Autodesk Fusion 360 part; units mm, degrees
sketch "Sketch1" plane through (0, 0, 0) normal (0, 0, 1) x (1, 0, 0)
  line L0 (-50, 0) -> (0, 0)
  line L1 (25, 25) -> (0, 0)
  line L2 (-50, 0) -> (-50, 140)
  line L3 (21.9831, 108.8475) -> (-62.7657, 108.8475)
  line L4 (-50, 108.8475) -> (-62.7657, 108.8475)
  line L5 (25, 25) -> (25, 110)
  line L6 (21.9831, 108.8475) -> (25, 108.8475)
extrude "Extrude1" add sketch "Sketch1" along normal blind 25
sketch "Sketch2" plane through (0, 0, 25) normal (0, 0, 1) x (-1, 0, 0)
  line L0 (-25, -108.8475) -> (50, -108.8475)
  line L1 (50, -108.8475) -> (50, 0)
  line L2 (50, 0) -> (0, 0)
  line L3 (0, 0) -> (-25, -25)
  line L4 (-25, -25) -> (-25, -108.8475)
sketch "Sketch3" plane through (0, 0, 25) normal (0, 0, 1) x (-1, 0, 0)
  line L0 (-10, -90) -> (-25, -97)
  line L1 (-25, -108.8475) -> (-25, -97)
  line L2 (-10, -90) -> (50, -90)
  line L3 (19.1012, -90) -> (19.1012, -70)
  line L4 (19.1012, -70) -> (40, -20)
  line L5 (40, -20) -> (40, 0)
  line L6 (40, 0) -> (50, 0)
  line L7 (50, 0) -> (50, -108.8475)
  line L8 (50, -90) -> (50, -108.8475)
  line L9 (-25, -97) -> (-25, -108.8475)
  line L10 (50, -108.8475) -> (50, -90)
  point P0 (-25, -108.8475)
  point P1 (50, 0)
  point P2 (50, -108.8475)
extrude "Extrude2" add sketch "Sketch3" along normal blind 16
sketch "Sketch4" plane through (0, 0, 25) normal (0, 0, 1) x (-1, 0, 0)
  line L0 (-10, -90) -> (-25, -100)
  line L1 (-25, -108.8475) -> (-25, -100)
  line L2 (-25, -108.8475) -> (50, -108.8475)
  line L3 (50, -108.8475) -> (50, -90)
  line L4 (50, -90) -> (-10, -90)
  point P0 (-25, -108.8475)
  point P1 (50, -108.8475)
extrude "Extrude3" add sketch "Sketch4" along normal blind 25
sketch "Sketch5" plane through (0, 0, 41) normal (0, 0, 1) x (-1, 0, 0)
  line L0 (19.1012, -90) -> (50, -90)
  line L1 (50, -90) -> (50, 0)
  line L2 (50, 0) -> (40, 0)
  line L3 (40, 0) -> (40, -20)
  line L4 (40, -20) -> (19.1012, -70)
  line L5 (19.1012, -70) -> (19.1012, -90)
  circle A0 centre (35, -75) radius 5
extrude "Extrude4" cut sketch "Sketch5" against normal blind 41 contours A0
sketch "Sketch6" plane through (0, 90, 0) normal (0, -1, 0) x (1, 0, 0)
  line L0 (-50, 41) -> (-19.1012, 41)
  line L1 (-19.1012, 41) -> (-19.1012, 25)
  line L2 (-19.1012, 25) -> (10, 25)
  line L3 (10, 25) -> (10, 50)
  line L4 (10, 50) -> (-50, 50)
  line L5 (-50, 50) -> (-50, 41)
  circle A0 centre (-10, 35) radius 5
  dimension "d11" = 10
extrude "Extrude5" cut sketch "Sketch6" against normal blind 25 contours A0
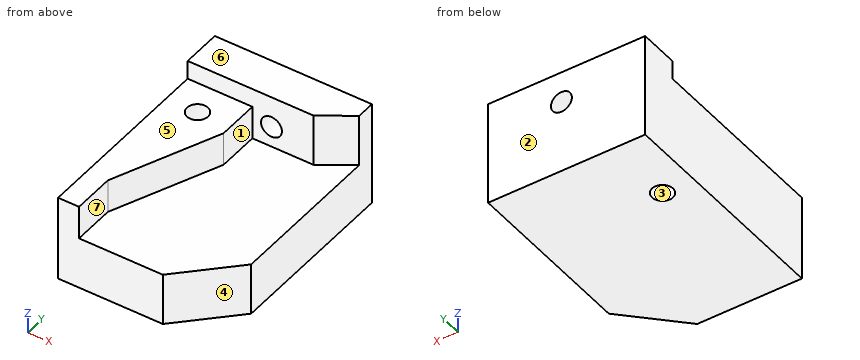
Read the model definition and answer for the solid it produces. Units are mm, in the model's axes. Face numbers are marked on the shaded views. A direction names the side the tool comes from. Round coordinates to 2 decimals unless told otherwise and drop trailing zeros. Loops run counter-clockwise (first coordinate to the right, second up) from the corner with the lowest first, then second, coordinate; pieces in that order, holes last. Notation, with made-up numbers: (-18.5, 6) -> (-7.5, 6) arc R35 cw to (-7.5, 43) -> close; hole circle Ø2 at (17, -3). An arc over 180 degrees is marked (long way). One line per item, written item: value.
1) The mould has two halves that part along Y. Classify the marked faces 1, 2, 3 and 4: pulls with the +Y half, pulls with the -Y half, needs draft (parallel to the pull), parting line crosses it, or undercut.
Answer list:
face 1: needs draft
face 2: pulls with the +Y half
face 3: undercut
face 4: pulls with the -Y half
2) For the marked faces 5, 6 and 7, determine the directions among +Z, -Z, +X, -X, +Y, -Y from which every point of the face is accessible in a straight line to the end or side of a thin tool.
Answer list:
face 5: +Z, +X, -X, -Y
face 6: +Z, +X, -X, +Y, -Y
face 7: +Z, +X, -Y
3) Consider L1, parallel to Y at x = -35, z = 23; L2, parallel to X at y = 75, z = 32; L3, parallel to Z at x = -10, y = 98. Determine where each line is inside the solid, lowest interval first. Write a range as [from, to].
Answer list:
L1: y = [0, 70], [80, 108.85]
L2: x = [-50, -40], [-30, -19.1]
L3: z = [0, 30], [40, 50]
4) A cutting plane is placed at B-B (x = -10). Determine the outline of the cut face in (y, z).
Answer list:
outline: (0, 0) -> (108.85, 0) -> (108.85, 30) -> (90, 30) -> (90, 25) -> (0, 25) -> close; (90, 40) -> (108.85, 40) -> (108.85, 50) -> (90, 50) -> close
5) A cutting plane is placed at C-C (z = 6.5). Determine the outline of the cut face in (x, y).
Answer list:
outline: (-50, 0) -> (0, 0) -> (25, 25) -> (25, 108.85) -> (-50, 108.85) -> close; hole circle Ø10 at (-35, 75)
6) A cutting plane is placed at D-D (x = 3). Determine the outline of the cut face in (y, z).
Answer list:
outline: (3, 0) -> (108.85, 0) -> (108.85, 50) -> (90, 50) -> (90, 25) -> (3, 25) -> close
7) Flat-ended cylindrical pins translate along their axes: P1, Ø6, axis at x = -23, y = 73.5, coming from the +Z side; P2, Ø1.5, axis at x = -18, y = 51.5, coming from the +Z side; P3, Ø10, axis at x = -19.5, y = 21.5, coming from the -Z side; P4, Ø13, axis at y = 76.5, z = 35, coming from the +X side. Find the tip coordinate at first contact, or state that the pin passes through.
Answer list:
P1: stops at z = 41
P2: stops at z = 25
P3: stops at z = 0
P4: stops at x = -19.1
8) A cutting plane is placed at A-A (y = 75). Determine the outline of the cut face in (x, z).
Answer list:
outline: (-50, 0) -> (-40, 0) -> (-40, 41) -> (-50, 41) -> close; (-30, 0) -> (25, 0) -> (25, 25) -> (-19.1, 25) -> (-19.1, 41) -> (-30, 41) -> close
